Read the model definition and answer for the solid it produces. Units are mm, in the model's axes. Coordinates: 2 decimals unless noted, no trailing zeros. Write each loop counter-clockwise with the first axis right and the second up, starting at its lowest first coordinate (ties: lowest second). Pieces come first, ordered by that corner, then holes.
(1) The part is cut by section C-C, the plane y = 4.25. Determine the outline of the cut face in (x, z), and give its area (3 significant figures).
(2) Straight lines are drawn through the part: line 1 along Z through (x, y) = (1.45, 0); line 2 along Z through (x, y) = (2.85, 1); line 3 along Y through (x, z) = (3.2, 1.25). For each, find the intervals that lie inside material, in ascending order.
(3) Given pin 1 (5.5 mm diameter, centred on y = 0, z = 0, fed in from +X); pin 2 (3 mm diameter, centred on x = 1.5, z = -3.5, fed in from -Y), each flat-ended and moving along its own axis, determine where each tip first touches the part or whether it passes through.
(4) The part is cut by section B-B, the plane x = 1.7. Determine the outline of the cut face in (y, z), and give its area (3 significant figures).
(5) Determine the mould class of faces 1 (the cylindrical face through (2.78, 3.32, 0.74)), 2 (the flat face through (6, -3, 3)), 3 (the flat face through (3, 0, 6)) for opening direction Z: pulls with the +Z half, pulls with the -Z half, needs draft (parallel to the pull), parting line crosses it, or undercut.
(6) The part is cut by section A-A, the plane y = 0. Determine the outline of the cut face in (x, z) (3 decimals), and give its area (3 significant figures).
```python
from build123d import *

# Parameters (mm, degrees)
EXTRUDE_1_DEPTH = 6


with BuildPart() as part:
    # 草图2 → 凸台-拉伸1 (new body)
    with BuildSketch(Plane(origin=(0, 0, 0), x_dir=(0, 0, -1), z_dir=(1, 0, 0))):
        Polygon((6, -3.464101615), (6, 3.464101615), (0, 6.92820323), (-6, 3.464101615), (-6, -3.464101615), (0, -6.92820323), align=None)
    extrude(amount=EXTRUDE_1_DEPTH)

    # 草图4 → M8 螺纹孔1 (revolve, cut)
    with BuildSketch(Plane(origin=(6, 0, 0), x_dir=(0, 0, -1), z_dir=(0, 1, 0))):
        Polygon((0, 0), (0, 6), (3.4, 6), (3.4, 0.524437269), (4.025, 0), align=None)
    revolve(axis=Axis((12.35, 0, 0), (-1, 0, 0)), mode=Mode.SUBTRACT)


solid = part.part
```
Computed:
1. outline: (0, -4.64) - (6, -4.64) - (6, 4.64) - (0, 4.64) - close
1. area: 55.7 mm2
2. line 1: z = -6 to -3.4, 3.4 to 6
2. line 2: z = -6 to -3.25, 3.25 to 6
2. line 3: y = -6.21 to -3.16, 3.16 to 6.21
3. pin 1: passes through
3. pin 2: stops at y = -5.77
4. outline: (-6.93, 0) - (-3.46, -6) - (3.46, -6) - (6.93, 0) - (3.46, 6) - (-3.46, 6) - close; hole circle Ø6.8 at (0, 0)
4. area: 88.4 mm2
5. face 1: undercut
5. face 2: needs draft
5. face 3: pulls with the +Z half
6. outline: (0, -6) - (6, -6) - (6, -4.025) - (5.476, -3.4) - (0, -3.4) - close; (0, 3.4) - (5.476, 3.4) - (6, 4.025) - (6, 6) - (0, 6) - close
6. area: 30.9 mm2
